Here's how the part is built. I have some questions about the finished solid (model axes, mm). Coordinates: 2 decimals unless noted, no trailing zeros. Loops run counter-clockwise (first coordinate to the right, second up) from the corner with the lowest first, then second, coordinate; pieces in that order, holes last.
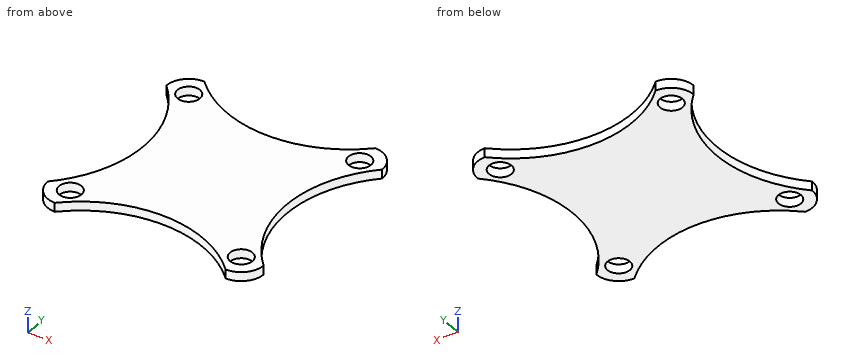
from build123d import *

# Parameters (mm, degrees)
MODEL_R             = 2.25
BOSS_EXTRUDE1_DEPTH = 1.8


with BuildPart() as part:
    # Model → Boss-Extrude1 (new body)
    with BuildSketch(Plane.XY):
        with BuildLine():
            ThreePointArc((-81.255144817, -18.241548457), (-64.020000155, -25.380579125), (-46.784855492, -18.241548457))
            ThreePointArc((-46.784855492, -18.241548457), (-43.586394524, -19.566394369), (-42.261548612, -22.764855338))
            ThreePointArc((-42.261548612, -22.764855338), (-49.40057928, -40), (-42.261548612, -57.235144662))
            ThreePointArc((-42.261548612, -57.235144662), (-43.586394524, -60.433605631), (-46.784855493, -61.758451543))
            ThreePointArc((-46.784855493, -61.758451543), (-64.020000155, -54.619420875), (-81.255144817, -61.758451543))
            ThreePointArc((-81.255144817, -61.758451543), (-84.453605786, -60.433605631), (-85.778451698, -57.235144662))
            ThreePointArc((-85.778451698, -57.235144662), (-78.639421029, -40), (-85.778451698, -22.764855338))
            ThreePointArc((-85.778451698, -22.764855338), (-84.453605786, -19.566394369), (-81.255144817, -18.241548457))
        make_face()
        with Locations((-81.264218317, -22.773928838)):
            Circle(MODEL_R, mode=Mode.SUBTRACT)
        with Locations((-81.246071317, -57.244218163)):
            Circle(MODEL_R, mode=Mode.SUBTRACT)
        with Locations((-46.775781992, -57.226071162)):
            Circle(MODEL_R, mode=Mode.SUBTRACT)
        with Locations((-46.793928993, -22.755781837)):
            Circle(MODEL_R, mode=Mode.SUBTRACT)
    extrude(amount=BOSS_EXTRUDE1_DEPTH)


solid = part.part
Q1. Suppose I cut it at C-C on y = -21.5. Write out the boundary of the cut face in (x, z).
Q2. Please list where these lines run through material, in increasing order: probe 1 along Y at (x, z) = (-47, 1.15); probe 2 along Y at (x, z) = (-83, 1.7); probe 3 along Y at (x, z) = (-75, 1.4).
Q3. Suppose I cut it at B-B on z = 0.65. Write out the boundary of the cut face in (x, y).
Q4. Will these pins go through, and if not, where does the flat tip stop? P1, Ø3.5, axis at x = -46.78, y = -57.23, coming from the -Z side; P2, Ø8, axis at x = -66.5, y = -55.5, coming from the -Z side.
Q5. Suppose I cut it at A-A on y = -58. Write out the boundary of the cut face in (x, z), and give its area (3 significant figures).
Q6. Suppose I cut it at D-D on x = -74.5. Write out the boundary of the cut face in (y, z), and give its area (3 significant figures).
Check values:
1. outline: (-85.6, 0) - (-83.12, 0) - (-83.12, 1.8) - (-85.6, 1.8) - close; (-79.41, 0) - (-77.22, 0) - (-77.22, 1.8) - (-79.41, 1.8) - close; (-50.82, 0) - (-48.66, 0) - (-48.66, 1.8) - (-50.82, 1.8) - close; (-44.93, 0) - (-42.44, 0) - (-42.44, 1.8) - (-44.93, 1.8) - close
2. probe 1: y = -61.55 to -59.46, -54.99 to -50.55, -29.45 to -25, -20.52 to -18.45
2. probe 2: y = -61.41 to -58.65, -55.83 to -53.91, -26.09 to -24.21, -21.34 to -18.59
2. probe 3: y = -57.23 to -22.77
3. outline: (-85.78, -57.24) arc R4.52 ccw to (-81.26, -61.76) arc R24.37 cw to (-46.78, -61.76) arc R4.52 ccw to (-42.26, -57.24) arc R24.37 cw to (-42.26, -22.76) arc R4.52 ccw to (-46.78, -18.24) arc R24.37 cw to (-81.26, -18.24) arc R4.52 ccw to (-85.78, -22.76) arc R24.37 cw to start; hole circle Ø4.5 at (-81.26, -22.77); hole circle Ø4.5 at (-81.25, -57.24); hole circle Ø4.5 at (-46.79, -22.76); hole circle Ø4.5 at (-46.78, -57.23)
4. P1: passes through
4. P2: stops at z = 0
5. outline: (-85.71, 0) - (-83.37, 0) - (-83.37, 1.8) - (-85.71, 1.8) - close; (-79.13, 0) - (-76.4, 0) - (-76.4, 1.8) - (-79.13, 1.8) - close; (-51.64, 0) - (-48.89, 0) - (-48.89, 1.8) - (-51.64, 1.8) - close; (-44.66, 0) - (-42.33, 0) - (-42.33, 1.8) - (-44.66, 1.8) - close
5. area: 18.3 mm2
6. outline: (-56.99, 0) - (-23.01, 0) - (-23.01, 1.8) - (-56.99, 1.8) - close
6. area: 61.2 mm2
